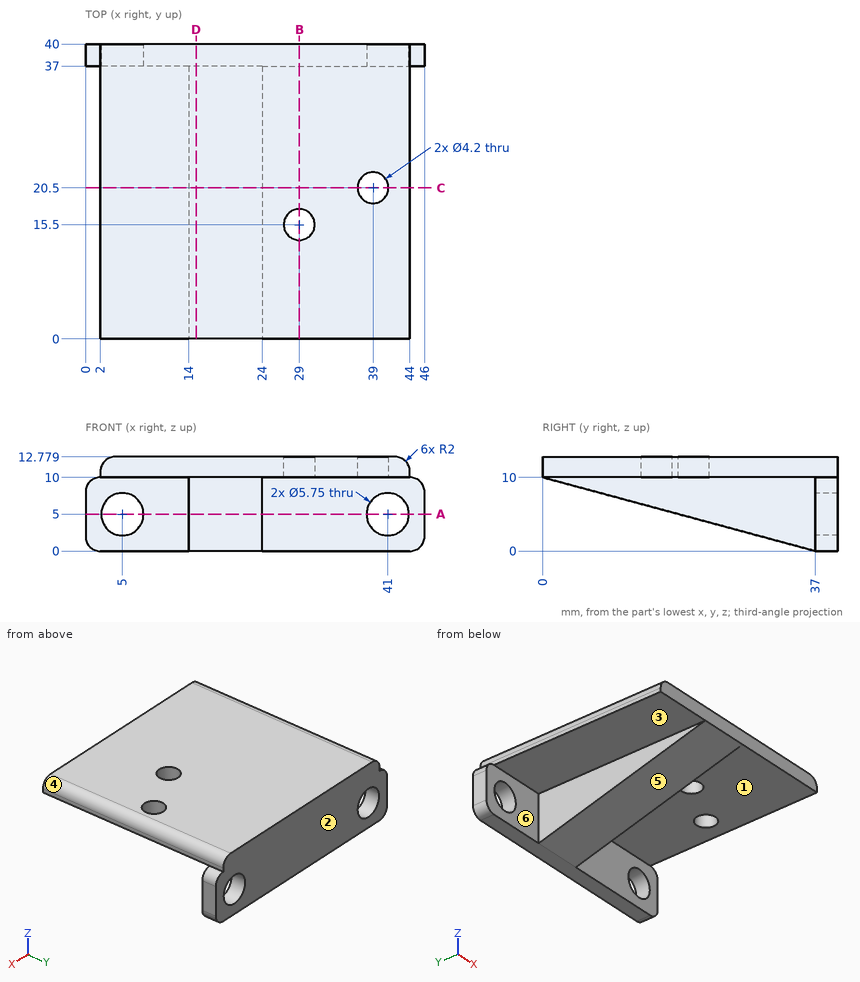
Design review of the part shown in the three views and the two pictorial views. Dimensions are in mm from the part's minimum x, y and z. A direction names the side the tool comes from. Round coordinates to 2 decimals unless told otherwise and drop trailing zeros. Write each loop counter-clockwise with the first axis right and the second up, starting at its lowest first coordinate (ties: lowest second). Pieces come first, ordered by that corner, then holes.
Item 1: Consider section D-D on x = 15. Give the boundary of the cut face in (y, z).
Item 2: For the marked faces 1, 2 and 3, list the 3-axis set-ups (+Z, -Z, +X, -X, +Y, -Y) from which the entire face can be reached by the end or side of a thin tool; tool diameter is ignored.
Item 3: Wall thickness on L1, parallel to Y at x = 39, z = 11.1; L2, parallel to Z at x = 41, y = 38.45 (1 decimal); L3, parallel to X at y = 38, z = 5.5: over which ranges is each line inside the solid? List them lowest first.
Item 4: Consider section A-A on z = 5. Give the boundary of the cut face in (x, y) (1 decimal).
Item 5: Consider section C-C on y = 20.5. Give the boundary of the cut face in (x, z).
Item 6: For pin 1 Ø9.5 at (x, y) = (10.5, 26) entering from -Z (1 decimal); pin 2 Ø0.6 at (y, z) = (13, 10.5) entering from +X; pin 3 Ø6 at (y, z) = (15, 3) entering from -X; pin 4 Ø3 at (y, z) = (13.5, 3) entering from +X, all flat-tipped, find the tip position at first contact; note any pin that passes through.
Item 7: Consider section B-B on x = 29. Give the boundary of the cut face in (y, z).
Item 8: Draft analysis for pull direction Z (two halves, no side actions). For the marked faces 4, 5 and 6, state which applies: released by +Z, released by -Z, zero draft, split by the parting line, or undercut.
Check values:
1. outline: (0, 10) - (37, 0) - (40, 0) - (40, 12.78) - (0, 12.78) - close
2. face 1: -Z, +X, -Y
2. face 2: +Z, -Z, +X, -X, +Y
2. face 3: -Z, -X, -Y
3. L1: y = 0 to 18.4, 22.6 to 40
3. L2: z = 0 to 2.1, 7.9 to 12.8
3. L3: x = 0 to 2.17, 7.83 to 38.17, 43.83 to 46
4. outline: (0, 37) - (2.1, 37) - (2.1, 40) - (0, 40) - close; (7.9, 37) - (14, 37) - (14, 18.5) - (24, 18.5) - (24, 37) - (38.1, 37) - (38.1, 40) - (7.9, 40) - close; (43.9, 37) - (46, 37) - (46, 40) - (43.9, 40) - close
5. outline: (2, 10) - (14, 10) - (14, 4.46) - (24, 4.46) - (24, 10) - (36.9, 10) - (36.9, 12.78) - (4, 12.78) arc R2 ccw to (2, 10.78) - close; (41.1, 10) - (44, 10) - (44, 10.78) arc R2 ccw to (42, 12.78) - (41.1, 12.78) - close
6. pin 1: stops at z = 2.1
6. pin 2: stops at x = 44
6. pin 3: stops at x = 14
6. pin 4: passes through
7. outline: (0, 10) - (13.4, 10) - (13.4, 12.78) - (0, 12.78) - close; (17.6, 10) - (37, 10) - (37, 0) - (40, 0) - (40, 12.78) - (17.6, 12.78) - close
8. face 4: released by +Z
8. face 5: released by -Z
8. face 6: zero draft
